Build history of the part. All positions in model axes, mm. A direction names the side the tool comes from. Coordinates: 2 decimals unless noted, no trailing zeros. Loops run counter-clockwise (first coordinate to the right, second up) from the corner with the lowest first, then second, coordinate; pieces in that order, holes last. Notation, with made-up numbers: M 18,56.5 L 70,56.5 A15 ccw 70,81.5 Z; hole C 1,40 d2. An arc over 180 degrees is marked long. Write each question's results on one line, items separated by ' | '. Start each with the question number.
from build123d import *

# Parameters (mm, degrees)
SKETCH1_R           = 12.5
SKETCH1_R_2         = 7.5005
BOSS_EXTRUDE1_DEPTH = 25
BOSS_EXTRUDE2_START = 25
SKETCH1_3_R         = 12.5
SKETCH1_3_R_2       = 7.5005
BOSS_EXTRUDE2_DEPTH = 2.5
BOSS_EXTRUDE5_DEPTH = 5
SKETCH3_R           = 13.462912018
BOSS_EXTRUDE6_DEPTH = 15
SKETCH4_R           = 7.5
BOSS_EXTRUDE7_DEPTH = 20


with BuildPart() as part:
    # Sketch1 → Boss-Extrude1 (new body)
    with BuildSketch(Plane(origin=(0, 0, 0), x_dir=(1, 0, 0), z_dir=(0, 1, 0))):
        Circle(SKETCH1_R)
        Circle(SKETCH1_R_2, mode=Mode.SUBTRACT)
    extrude(amount=BOSS_EXTRUDE1_DEPTH)

    # Sketch1<3> → Boss-Extrude2 (add)
    with BuildSketch(Plane(origin=(0, 0, 0), x_dir=(1, 0, 0), z_dir=(0, 1, 0)).offset(BOSS_EXTRUDE2_START)):
        Circle(SKETCH1_3_R)
        Circle(SKETCH1_3_R_2, mode=Mode.SUBTRACT)
        Circle(SKETCH1_3_R_2)
    extrude(amount=BOSS_EXTRUDE2_DEPTH)

    # Sketch2 → Boss-Extrude5 (add, symmetric)
    with BuildSketch(Plane(origin=(0, 0, 0), x_dir=(0, 0, -1), z_dir=(1, 0, 0))):
        with BuildLine():
            Line((110, 45.5), (85, 45.5))
            add(Edge.make_bspline(
                [(0, 27.5), (27.318342435, 39.481167594), (59.380064257, 28.466617173), (85, 45.5)],
                knots=[0, 0, 0, 0, 1, 1, 1, 1], degree=3))
            Line((0, 27.5), (10.078558278, 27.5))
            Line((10.078558278, 27.5), (10.078558278, 6.752961332))
            add(Edge.make_bspline(
                [(10.078558278, 6.752961332), (40.207506706, 28.515228395), (81.426628227, 21.377572534), (110, 45.5)],
                knots=[0, 0, 0, 0, 1, 1, 1, 1], degree=3))
        make_face()
    extrude(amount=BOSS_EXTRUDE5_DEPTH, both=True)

    # Sketch3 → Boss-Extrude6 (add)
    with BuildSketch(Plane(origin=(0, 45.5, 0), x_dir=(1, 0, 0), z_dir=(0, 1, 0))):
        with Locations((0, 97.5)):
            Circle(SKETCH3_R)
    extrude(amount=-BOSS_EXTRUDE6_DEPTH)

    # Sketch4 → Boss-Extrude7 (add)
    with BuildSketch(Plane(origin=(0, 45.5, 0), x_dir=(1, 0, 0), z_dir=(0, 1, 0))):
        with Locations((0, 97.5)):
            Circle(SKETCH4_R)
    extrude(amount=BOSS_EXTRUDE7_DEPTH)


solid = part.part
1. Mould opens along X. For faces 1 (the flat face through (0, 27.5, 3)), 2 (the cylindrical face through (7.154, 12.325, -2.253)), 3 (the flat face through (0, 25, 0)), 4 (the cylindrical face through (5.77, 13.56, 11.09)) say: +X half, -X half, draft (parallel to the pull), parting line (faces both ways), or undercut.
2. Pin check, flat tips, straight feed: pin 1 (3 mm diameter, centred on x = -7.5, y = 48, fed in from -Z); pin 2 (10 mm diameter, centred on x = -10.5, y = 55, fed in from -Z); pin 3 (5 mm diameter, centred on x = -6.5, y = 45, fed in from -Z). Stop position of each tip, or through.
3. Band-saw the part on B-B, the plane x = -9. List the corners of the cut face in (y, z).
4. Which spindle directions (+Z, -Z, +X, -X, +Y, -Y) get a long thin tool onto all of the face, cutting with end or side? Do faces 5 (the flat face through (6, 45.5, -92)), 6 (the flat face through (0, 0, 8)), 7 (the flat face through (0, 30.5, -98)). Say none if no direction does.
5. Band-saw the part on A-A, the plane z = -97.5. List the corners of the cut face in (x, y).
6. Band-saw the part on C-C, the plane x = 10.25. List the corners of the cut face in (y, z).
7. Wall check: line 1 along X through (y, z) = (5, 0); line 2 along X through (y, z) = (22.5, -42). Give the ranges that are in metal, low to high.
Checked values:
1) face 1: draft | face 2: undercut | face 3: undercut | face 4: parting line
2) pin 1: z = -102 | pin 2: z = -102.6 | pin 3: z = -110.35
3) outline: M 0,-8.67 L 27.5,-8.67 L 27.5,8.67 L 0,8.67 Z; M 30.5,-107.51 L 45.5,-107.51 L 45.5,-87.49 L 30.5,-87.49 Z
4) face 5: +Y | face 6: +Z, -Z, +X, -X, -Y | face 7: -Z, +X, -X, -Y
5) outline: M -13.46,30.5 L 13.46,30.5 L 13.46,45.5 L 7.5,45.5 L 7.5,65.5 L -7.5,65.5 L -7.5,45.5 L -13.46,45.5 Z
6) outline: M 0,-7.15 L 27.5,-7.15 L 27.5,7.15 L 0,7.15 Z; M 30.5,-106.23 L 45.5,-106.23 L 45.5,-88.77 L 30.5,-88.77 Z
7) line 1: -12.5 to -7.5, 7.5 to 12.5 | line 2: -5 to 5
